Geometry: final body of the model. Coordinates: model frame, mm. Give positions to 0.01 mm unless a question says otherwise; leave off trailing zeros. Write each loop counter-clockwise with the first axis right and the second up, starting at its lowest first coordinate (ties: lowest second). Pieces come first, ordered by that corner, then holes.
Q1. Pin query (flat end, axial travel): pin 1 (2 mm diameter, centred on x = 42.5, z = 1, fed in from +Y); pin 2 (2.5 mm diameter, centred on y = -113.5, z = 3.5, fed in from -X); pin 3 (1.5 mm diameter, centred on x = 230.5, z = 2, fed in from -Y); pin 4 (1.8 mm diameter, centred on x = 185.92, y = -5, fed in from -Z). Return the tip coordinate at first contact, or that it passes through.
Q2. Line query: L1, parallel to Y at x = 220, z = 3.3; L2, parallel to X at y = -96, z = 4.55; L3, parallel to Y at x = 138.5, z = 4.65. Output: solid intervals per line, ascending.
Q3. Cut plane D-D on y = -138.5. Return the cut outline in (x, z).
Q4. Draft query along X for faces 1 (the face through (101.38, -212.902, 2.465)), 2 (the face through (151, -122, 5)), 3 (the face through (218.37, -37.32, 2.54)), 4 (the face through (246.99, -67.15, 2.46)). Return one class per face: pulls with the +X half, pulls with the -X half, needs draft (parallel to the pull), parting line crosses it, or undercut.
Q5. Cut plane C-C on x = 122.5. Return the cut outline in (y, z).
Q6. Cut plane A-A on z = 1.7. Return the cut outline in (x, y), plus the area to 3 significant figures.
Q7. Cut plane B-B on y = -30. Return the cut outline in (x, z).
```python
from build123d import *

# Parameters (mm, degrees)
EXTRUDE_1_DEPTH     = 5
SKETCH_2_R          = 7.5
CUT_EXTRUDE_1_DEPTH = 5
SKETCH_3_W          = 5
SKETCH_3_H          = 6
CUT_EXTRUDE_3_DEPTH = 51
CUT_EXTRUDE_4_REACH = 353.474
CUT_EXTRUDE_6_REACH = 353.474
SKETCH_6_R          = 1.5
CUT_EXTRUDE_7_REACH = 353.474
SKETCH_7_W          = 51
SKETCH_7_H          = 217.5
CUT_EXTRUDE_9_DEPTH = 10


with BuildPart() as part:
    # 草图1 → 凸台-拉伸1 (new body)
    with BuildSketch(Plane.XY):
        with BuildLine():
            Line((210, -247), (210, -237))
            Line((210, -237), (210, -70))
            Line((210, -70), (210, 0))
            Line((210, 0), (10, 0))
            ThreePointArc((10, 0), (2.928932188, -2.928932188), (0, -10))
            Line((0, -10), (0, -237))
            Line((0, -237), (0, -247))
            Line((0, -247), (10, -247))
            Line((10, -247), (200, -247))
            Line((200, -247), (210, -247))
        make_face()
        with BuildLine():
            Line((210, 0), (210, -70))
            Line((210, -70), (240, -70))
            ThreePointArc((240, -70), (247.071067812, -67.071067812), (250, -60))
            Line((250, -60), (250, -10))
            ThreePointArc((250, -10), (247.071067812, -2.928932188), (240, 0))
            Line((240, 0), (210, 0))
        make_face()
    extrude(amount=EXTRUDE_1_DEPTH)

    # 草图2 → 切除-拉伸1 (cut)
    with BuildSketch(Plane.XY.offset(5)):
        with Locations((220, -30)):
            Circle(SKETCH_2_R)
    extrude(amount=-CUT_EXTRUDE_1_DEPTH, mode=Mode.SUBTRACT)

    # 草图3 → 切除-拉伸3 (cut)
    with BuildSketch(Plane.ZY):
        with Locations((2.5, -214.5)):
            Rectangle(SKETCH_3_W, SKETCH_3_H)
    extrude(amount=-CUT_EXTRUDE_3_DEPTH, mode=Mode.SUBTRACT)

    # 草图4 → 切除-拉伸4 (cut, up to next)
    with BuildSketch(Plane.XY.offset(5), mode=Mode.PRIVATE) as cut_extrude_4_sk1:
        with BuildLine():
            Line((51, -211.5), (51, -217.5))
            ThreePointArc((51, -217.5), (54, -214.5), (51, -211.5))
        make_face()
    cut_extrude_4_tool1 = extrude(cut_extrude_4_sk1.sketch, amount=-CUT_EXTRUDE_4_REACH, mode=Mode.PRIVATE) & part.part
    add(cut_extrude_4_tool1.solids().sort_by_distance((52.27324, -214.5, 5))[0], mode=Mode.SUBTRACT)

    # 草图6 → 切除-拉伸6 (cut, up to next)
    with BuildSketch(Plane.XY.offset(5), mode=Mode.PRIVATE) as cut_extrude_6_sk1:
        with Locations((218.076993274, -5)):
            Circle(SKETCH_6_R)
    cut_extrude_6_tool1 = extrude(cut_extrude_6_sk1.sketch, amount=-CUT_EXTRUDE_6_REACH, mode=Mode.PRIVATE) & part.part
    # 草图6 → 切除-拉伸6 (cut, up to next)
    with BuildSketch(Plane.XY.offset(5), mode=Mode.PRIVATE) as cut_extrude_6_sk2:
        with Locations((185.921620837, -5)):
            Circle(SKETCH_6_R)
    cut_extrude_6_tool2 = extrude(cut_extrude_6_sk2.sketch, amount=-CUT_EXTRUDE_6_REACH, mode=Mode.PRIVATE) & part.part
    add(cut_extrude_6_tool1.solids().sort_by_distance((218.076993, -5, 5))[0], mode=Mode.SUBTRACT)
    add(cut_extrude_6_tool2.solids().sort_by_distance((185.921621, -5, 5))[0], mode=Mode.SUBTRACT)

    # 草图7 → 切除-拉伸7 (cut, up to next)
    with BuildSketch(Plane.XY.offset(5), mode=Mode.PRIVATE) as cut_extrude_7_sk1:
        with Locations((25.5, -108.75)):
            Rectangle(SKETCH_7_W, SKETCH_7_H)
    cut_extrude_7_tool1 = extrude(cut_extrude_7_sk1.sketch, amount=-CUT_EXTRUDE_7_REACH, mode=Mode.PRIVATE) & part.part
    add(cut_extrude_7_tool1.solids().sort_by_distance((25.5, -108.75, 5))[0], mode=Mode.SUBTRACT)

    # 草图8 → 切除-拉伸9 (cut)
    with BuildSketch(Plane(origin=(0, 0, 0), x_dir=(-1, 0, 0), z_dir=(0, 0, -1))):
        with BuildLine():
            Line((-66, -234), (-66, -184.298412176))
            ThreePointArc((-66, -184.298412176), (-101.923530523, -213.253778558), (-143.136484598, -234))
            Line((-143.136484598, -234), (-66, -234))
        make_face()
    extrude(amount=-CUT_EXTRUDE_9_DEPTH, mode=Mode.SUBTRACT)


solid = part.part
```
Data:
1. pin 1: stops at y = -217.5
1. pin 2: stops at x = 51
1. pin 3: stops at y = -70
1. pin 4: passes through
2. L1: y = -70 to -37.5, -22.5 to 0
2. L2: x = 51 to 210
2. L3: y = -247 to -234, -232.19 to 0
3. outline: (51, 0) - (210, 0) - (210, 5) - (51, 5) - close
4. face 1: undercut
4. face 2: needs draft
4. face 3: undercut
4. face 4: pulls with the +X half
5. outline: (-247, 0) - (-234, 0) - (-234, 5) - (-247, 5) - close; (-224.98, 0) - (0, 0) - (0, 5) - (-224.98, 5) - close
6. outline: (0, -247) - (210, -247) - (210, -70) - (240, -70) arc R10 ccw to (250, -60) - (250, -10) arc R10 ccw to (240, 0) - (51, 0) - (51, -211.5) arc R3 cw to (51, -217.5) - (0, -217.5) - close; hole (66, -234) - (143.14, -234) arc R218 cw to (66, -184.3) - close; hole circle Ø3 at (185.92, -5); hole circle Ø15 at (220, -30); hole circle Ø3 at (218.08, -5)
6. area: 41,700 mm2
7. outline: (51, 0) - (212.5, 0) - (212.5, 5) - (51, 5) - close; (227.5, 0) - (250, 0) - (250, 5) - (227.5, 5) - close
